from build123d import *

# Parameters (mm, degrees)
SKETCH1_W           = 27
SKETCH1_H           = 26
BOSS_EXTRUDE1_DEPTH = 15
CUT_EXTRUDE2_DEPTH  = 23.5
SKETCH5_W           = 3.601284645
SKETCH5_H           = 15
CUT_EXTRUDE3_DEPTH  = 33.912763482
SKETCH6_R           = 3
CUT_EXTRUDE4_DEPTH  = 33.912763482
SKETCH11_R          = 4.875
CUT_EXTRUDE6_DEPTH  = 25.005207768
SKETCH13_W          = 26
SKETCH13_H          = 15
BOSS_EXTRUDE3_DEPTH = 15
SKETCH14_W          = 5
SKETCH14_H          = 26
BOSS_EXTRUDE4_DEPTH = 20
SKETCH15_R          = 3
CUT_EXTRUDE7_DEPTH  = 20
BOSS_EXTRUDE5_DEPTH = 3
BOSS_EXTRUDE6_DEPTH = 3


with BuildPart() as part:
    # Sketch1 → Boss-Extrude1 (new body)
    with BuildSketch(Plane(origin=(0, 0, 0), x_dir=(1, 0, 0), z_dir=(0, 1, 0))):
        Rectangle(SKETCH1_W, SKETCH1_H)
    extrude(amount=BOSS_EXTRUDE1_DEPTH)

    # Sketch4 → Cut-Extrude2 (cut)
    with BuildSketch(Plane(origin=(13.5, 0, 0), x_dir=(0, 0, -1), z_dir=(1, 0, 0))):
        Polygon((-10, 2), (-7.5, 2), (-7.5, 0), (7.5, 0), (7.5, 2), (10, 2), (10, 8), (7.5, 8), (7.5, 10), (-7.5, 10), (-7.5, 8), (-10, 8), align=None)
    extrude(amount=-CUT_EXTRUDE2_DEPTH, mode=Mode.SUBTRACT)

    # Sketch5 → Cut-Extrude3 (cut, through all)
    with BuildSketch(Plane(origin=(0, 0, -13), x_dir=(-1, 0, 0), z_dir=(0, 0, -1))):
        with Locations((-11.699357678, 7.5)):
            Rectangle(SKETCH5_W, SKETCH5_H)
    extrude(amount=-CUT_EXTRUDE3_DEPTH, mode=Mode.SUBTRACT)

    # Sketch6 → Cut-Extrude4 (cut, through all)
    with BuildSketch(Plane(origin=(0, 0, -13), x_dir=(-1, 0, 0), z_dir=(0, 0, -1))):
        with Locations((0, 5)):
            Circle(SKETCH6_R)
    extrude(amount=-CUT_EXTRUDE4_DEPTH, mode=Mode.SUBTRACT)

    # Sketch11 → Cut-Extrude6 (cut, through all)
    with BuildSketch(Plane(origin=(0, 15, 0), x_dir=(1, 0, 0), z_dir=(0, 1, 0))):
        with Locations(Location((0, 0, 0), (0, 0, 270))):
            Circle(SKETCH11_R)
    extrude(amount=-CUT_EXTRUDE6_DEPTH, mode=Mode.SUBTRACT)

    # Sketch13 → Boss-Extrude3 (add)
    with BuildSketch(Plane.ZY.offset(13.5)):
        with Locations((0, 7.5)):
            Rectangle(SKETCH13_W, SKETCH13_H)
    extrude(amount=BOSS_EXTRUDE3_DEPTH)

    # Sketch14 → Boss-Extrude4 (add)
    with BuildSketch(Plane(origin=(0, 15, 0), x_dir=(1, 0, 0), z_dir=(0, 1, 0))):
        with Locations((-26, 0)):
            Rectangle(SKETCH14_W, SKETCH14_H)
    extrude(amount=BOSS_EXTRUDE4_DEPTH)

    # Sketch15 → Cut-Extrude7 (cut)
    with BuildSketch(Plane(origin=(-23.5, 0, 0), x_dir=(0, 0, -1), z_dir=(1, 0, 0))):
        with Locations((0, 25)):
            Circle(SKETCH15_R)
    extrude(amount=-CUT_EXTRUDE7_DEPTH, mode=Mode.SUBTRACT)

    # Sketch16 → Boss-Extrude5 (add)
    with BuildSketch(Plane(origin=(0, 0, -13), x_dir=(-1, 0, 0), z_dir=(0, 0, -1))):
        Polygon((23.5, 35), (6.800642322, 15), (23.5, 15), align=None)
    extrude(amount=-BOSS_EXTRUDE5_DEPTH)

    # Sketch17 → Boss-Extrude6 (add)
    with BuildSketch(Plane.XY.offset(13)):
        Polygon((-23.5, 35), (-6.800642322, 15), (-23.5, 15), align=None)
    extrude(amount=-BOSS_EXTRUDE6_DEPTH)


solid = part.part
CAD build for the part. Positions are in the model's coordinates, mm. A direction names the side the tool comes from. Give positions to 0.01 mm unless a question says otherwise; leave off trailing zeros. Write each loop counter-clockwise with the first axis right and the second up, starting at its lowest first coordinate (ties: lowest second). Pieces come first, ordered by that corner, then holes. Notation, with made-up numbers: (49.25, 45) -> (69.25, 45) arc R25 ccw to (69.25, 83) -> close; hole circle Ø4 at (-6.75, 68). An arc over 180 degrees is marked (long way). Return JSON: item names as keys, results as strings.
Item 1: Band-saw the part on B-B (z = 0). List the corners of the cut face in (x, y) (3 decimals), then the cut area to 3 significant figures.
Answer below:
{"outline": "(-28.5, 0) -> (-10, 0) -> (-10, 10) -> (-4.875, 10) -> (-4.875, 15) -> (-23.5, 15) -> (-23.5, 22) -> (-28.5, 22) -> close; (-28.5, 28) -> (-23.5, 28) -> (-23.5, 35) -> (-28.5, 35) -> close; (4.875, 10) -> (9.899, 10) -> (9.899, 15) -> (4.875, 15) -> close", "area": "398 mm2"}
Item 2: Drill centre lines: probe 1 along Y at (x, z) = (-24.55, 0); probe 2 along X at (y, z) = (5, -10.75); probe 3 along Y at (x, z) = (0, -12.4). Where is each one in solid material? Low to high.
Answer below:
{"probe 1": "y = 0 to 22, 28 to 35", "probe 2": "x = -28.5 to -3, 3 to 9.9", "probe 3": "y = 0 to 2, 8 to 15"}
Item 3: Band-saw the part on C-C (z = 10.75). List the corners of the cut face in (x, y).
Answer below:
{"outline": "(-28.5, 0) -> (9.9, 0) -> (9.9, 15) -> (-6.8, 15) -> (-23.5, 35) -> (-28.5, 35) -> close; hole circle Ø6 at (0, 5)"}
Item 4: Band-saw the part on A-A (y = 5). List the corners of the cut face in (x, z), then the cut area to 3 significant figures.
Answer below:
{"outline": "(-28.5, -13) -> (-3, -13) -> (-3, -10) -> (-10, -10) -> (-10, 10) -> (-3, 10) -> (-3, 13) -> (-28.5, 13) -> close; (3, -13) -> (9.9, -13) -> (9.9, -10) -> (3, -10) -> close; (3, 10) -> (9.9, 10) -> (9.9, 13) -> (3, 13) -> close", "area": "564 mm2"}
Item 5: Band-saw the part on D-D (x = 6.5). List the corners of the cut face in (y, z), then the cut area to 3 significant figures.
Answer below:
{"outline": "(0, -13) -> (15, -13) -> (15, 13) -> (0, 13) -> (0, 7.5) -> (2, 7.5) -> (2, 10) -> (8, 10) -> (8, 7.5) -> (10, 7.5) -> (10, -7.5) -> (8, -7.5) -> (8, -10) -> (2, -10) -> (2, -7.5) -> (0, -7.5) -> close", "area": "210 mm2"}
Item 6: Two-plate mould, pull along Z, no slides. Class faces 1 (the flat face through (-15.267, 25.14, 11.521)), 2 (the flat face through (-13, 14, 13)), 3 (the flat face through (-19, 21, 10)): +Z half, -Z half, draft (parallel to the pull), parting line (faces both ways), or undercut.
Answer below:
{"face 1": "draft", "face 2": "+Z half", "face 3": "undercut"}
Item 7: Drop flat-ended pins along their axis: pin 1 (7 mm diameter, centred on x = 0, y = 5, fed in from -Z); pin 2 (5 mm diameter, centred on x = -11.5, z = 5.5, fed in from +Y); pin 3 (11 mm diameter, centred on x = 0, z = 0, fed in from -Y). Give the stop position or say it passes through.
Answer below:
{"pin 1": "stops at z = -13", "pin 2": "stops at y = 15", "pin 3": "stops at y = 10"}
Item 8: Tool access for faces 4 (the flat face through (6, 5, -10)), 5 (the flat face through (0.1, 10, -5.1)), 6 (the flat face through (-23.5, 22.6, 2.4)): list every direction of +Z, -Z, +X, -X, +Y, -Y with a clear straight run to the whole face (end or side of a thin tool).
Answer below:
{"face 4": "+X", "face 5": "+X, -Y", "face 6": "+X, +Y"}
